```python
from build123d import *


with BuildPart() as part:
    # 草图1 → 旋转1 (revolve)
    with BuildSketch(Plane.XY):
        with BuildLine():
            Line((-10.1, 0.5), (-5.873607887, 0.5))
            Line((-5.873607887, 0.5), (-5.584932753, 1))
            Line((-5.584932753, 1), (-5.084932753, 1))
            Line((-5.084932753, 1), (-4.432451432, 4.700405452))
            ThreePointArc((-4.432451432, 4.700405452), (-4.867701612, 5.044870418), (-4.632451432, 5.547619048))
            Line((-4.632451432, 5.547619048), (-4.632451432, 6.404761905))
            Line((-4.632451432, 6.404761905), (-3.680070479, 6.404761905))
            Line((-3.680070479, 6.404761905), (-3, 5.928571429))
            Line((-3, 5.928571429), (-3.251895687, 4.5))
            Line((-3.251895687, 4.5), (-3.960075014, 4.5))
            Line((-3.960075014, 4.5), (-4.753546427, 0))
            Line((-4.753546427, 0), (-10.5, 0))
            Line((-10.5, 0), (-11, 0.5))
            Line((-11, 0.5), (-11, 7))
            Line((-11, 7), (-10.5, 7))
            Line((-10.5, 7), (-10.5, 0.9))
            Line((-10.5, 0.9), (-10.1, 0.5))
        make_face()
    revolve(axis=Axis((0, 5.836193369, 0), (0, -1, 0)))


solid = part.part
```
Check sheet for the modelled part. Datum: model origin and axes. Units: mm. A direction names the side the tool comes from. Give positions to 0.01 mm unless a question says otherwise; leave off trailing zeros. Order: outer loops, then holes, each group sorted by start corner. A loop starts at its lowest first (then second) coordinate and runs counter-clockwise, first axis right, second up. Notation, with made-up numbers: M 18.25,80 L 56.25,80 A20 cw 56.25,119 Z; hole C -31.5,-37.75 d8. An arc over 180 degrees is marked long. Answer in a Markdown table with one row per item. Add a question column.
Q1. Release check for a two-part mould opening along X. For faces 4 (the flat face through (5, 0, 2)), 5 (the cylindrical face through (2.38, 3.8, 10.74)), 6 (the flat face through (-2, 1, 5)), 7 (the conical face through (-2.903, 5.68, -0.914)) record: released by +X, released by -X, zero draft, split by the parting line, or undercut.
Q2. Sectioned sample at C-C, the plane y = 5.25. Record the boundary of the cut face in (x, z), and give its area (3 significant figures).
Q3. Gauge pin test, flat ends, axial feed: pin 1 Ø8 at (x, z) = (-1, -4) entering from -Y; pin 2 Ø9 at (x, z) = (1, 0.5) entering from +Y; pin 3 Ø1 at (x, y) = (6.5, 1) entering from -Z; pin 4 Ø2 at (x, y) = (5, 1) entering from -Z. Record the tip position at first contact, or that the pin passes through.
Q4. Access from +Z, -Z, +X, -X, +Y, -Y to the whole of each face (thin tool, end or side, straight path). Record for faces 1 (the flat face through (-10, 7, 4)), 2 (the flat face through (-4.3, 0.5, 4.3)), 3 (the conical face through (3.66, 3.7, 2.8)).
Q5. Thickness scan on L1, parallel to X at y = 3, z = 0; L2, parallel to X at y = 6, z = 4; L3, parallel to Z at x = -1, y = 6. Record the ranges inside material, lowest first.
Verdict:
| question | item | result |
|---|---|---|
| 1 | face 4 | zero draft |
| 1 | face 5 | split by the parting line |
| 1 | face 6 | undercut |
| 1 | face 7 | undercut |
| 2 | outline | C 0,0 d22; C 0,0 d9.74; hole C 0,0 d21; hole C 0,0 d6.24 |
| 2 | area | 77.6 mm² |
| 3 | pin 1 | y = 0 |
| 3 | pin 2 | y = 6.4 |
| 3 | pin 3 | z = -9.22 |
| 3 | pin 4 | z = -10.25 |
| 4 | face 1 | +Z, -Z, +X, -X, +Y |
| 4 | face 2 | +Y |
| 4 | face 3 | none |
| 5 | L1 | -11 to -10.5, -4.73 to -4.22, 4.22 to 4.73, 10.5 to 11 |
| 5 | L2 | -10.25 to -9.71, -2.34 to 2.34, 9.71 to 10.25 |
| 5 | L3 | -10.95 to -10.45, -4.52 to -2.94, 2.94 to 4.52, 10.45 to 10.95 |
